The listing builds one solid part. Answer for the finished solid, in the listing's coordinates (mm). Round coordinates to 2 decimals unless told otherwise and drop trailing zeros. Write each loop counter-clockwise with the first axis right and the second up, starting at its lowest first coordinate (ties: lowest second). Pieces come first, ordered by that corner, then holes. Notation, with made-up numbers: M -23,-2 L 2,-2 A12 ccw 2,7 Z; hole C -9.5,4.25 d6. An arc over 180 degrees is marked long. Write each question's results on one line, items separated by ' | '.
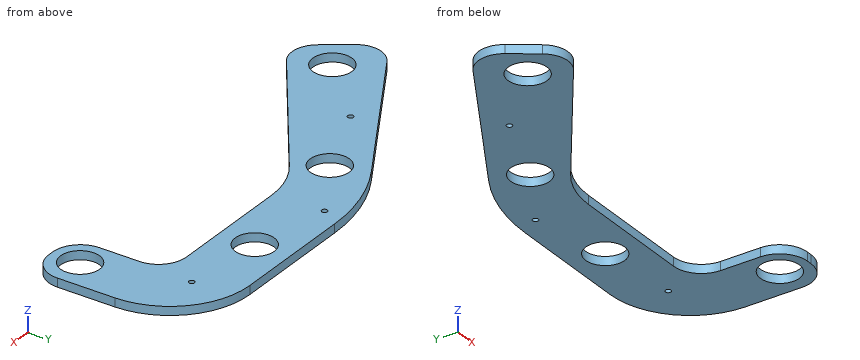
from build123d import *

# Parameters (mm, degrees)
BOSS_EXTRUDE1_DEPTH = 3.175
FILLET4_R           = 127
FILLET8_R           = 6.35
SKETCH4_R           = 14.2875
SKETCH4_R_2         = 2.032
CUT_EXTRUDE1_DEPTH  = 18.415
FILLET20_R          = 33.02
BOSS_EXTRUDE3_DEPTH = 6.35
FILLET23_R          = 127
FILLET24_R          = 19.05
FILLET25_R          = 19.05
SKETCH4_2_R         = 14.2875
SKETCH4_2_R_2       = 2.032
CUT_EXTRUDE2_DEPTH  = 6.35
FILLET27_R          = 60.96
FILLET28_R          = 20.32
FILLET29_R          = 20.32
FILLET30_R          = 20.32
FILLET31_R          = 58.42


with BuildPart() as part:
    # Sketch1 → Boss-Extrude1 (new body)
    with BuildSketch(Plane.XY):
        Polygon((0, 0), (-134.680588616, -95.49423569), (-170.699937974, -44.69423569), (-8.460282393, 50.869520386), (174.726114012, 50.869520386), (174.726114012, -31.75), (174.726114012, -69.85), (130.175, -69.85), (130.175, 0), align=None)
    extrude(amount=BOSS_EXTRUDE1_DEPTH)

    # Fillet4
    fillet4_edges = [part.edges().sort_by_distance(p)[0] for p in [
        (-8.460282393, 50.869520386, 1.5875),
    ]]
    fillet(fillet4_edges, radius=FILLET4_R)

    # Fillet8
    fillet8_edges = [part.edges().sort_by_distance(p)[0] for p in [
        (174.726114012, 50.869520386, 1.5875),
    ]]
    fillet(fillet8_edges, radius=FILLET8_R)

    # Sketch4 → Cut-Extrude1 (cut)
    with BuildSketch(Plane(origin=(0, 0, 0), x_dir=(-1, 0, 0), z_dir=(0, 0, -1))):
        with Locations((-151.503295524, -49.024477041)):
            Circle(SKETCH4_R)
        with Locations((130.843837195, -58.984690885)):
            Circle(SKETCH4_R)
        with Locations((30.055030467, 8.563007376)):
            Circle(SKETCH4_R)
        with Locations((-74.112358802, 25.4)):
            Circle(SKETCH4_R)
        with Locations((85.728358398, -14.612108422)):
            Circle(SKETCH4_R_2)
        with Locations((-132.677584994, 19.676786483)):
            Circle(SKETCH4_R_2)
        with Locations((-16.730295544, 36.917955745)):
            Circle(SKETCH4_R_2)
    extrude(amount=-CUT_EXTRUDE1_DEPTH, mode=Mode.SUBTRACT)

    # Fillet20
    fillet20_edges = [part.edges().sort_by_distance(p)[0] for p in [
        (-134.680588616, -95.49423569, 1.5875),
    ]]
    fillet(fillet20_edges, radius=FILLET20_R)

    # Sketch1<3> → Boss-Extrude3 (add)
    with BuildSketch(Plane.XY):
        Polygon((0, 0), (-134.680588616, -95.49423569), (-170.699937974, -44.69423569), (-8.460282393, 50.869520386), (174.726114012, 50.869520386), (174.726114012, -31.75), (174.726114012, -69.85), (130.175, -69.85), (130.175, 0), align=None)
    extrude(amount=BOSS_EXTRUDE3_DEPTH)

    # Fillet23
    fillet23_edges = [part.edges().sort_by_distance(p)[0] for p in [
        (-8.460282393, 50.869520386, 3.175),
    ]]
    fillet(fillet23_edges, radius=FILLET23_R)

    # Fillet24
    fillet24_edges = [part.edges().sort_by_distance(p)[0] for p in [
        (-170.699937974, -44.69423569, 3.175),
    ]]
    fillet(fillet24_edges, radius=FILLET24_R)

    # Fillet25
    fillet25_edges = [part.edges().sort_by_distance(p)[0] for p in [
        (-134.680588616, -95.49423569, 3.175),
    ]]
    fillet(fillet25_edges, radius=FILLET25_R)

    # Sketch4<2> → Cut-Extrude2 (cut)
    with BuildSketch(Plane(origin=(0, 0, 0), x_dir=(-1, 0, 0), z_dir=(0, 0, -1))):
        with Locations((-151.503295524, -49.024477041)):
            Circle(SKETCH4_2_R)
        with Locations((130.843837195, -58.984690885)):
            Circle(SKETCH4_2_R)
        with Locations((30.055030467, 8.563007376)):
            Circle(SKETCH4_2_R)
        with Locations((-74.112358802, 25.4)):
            Circle(SKETCH4_2_R)
        with Locations((85.728358398, -14.612108422)):
            Circle(SKETCH4_2_R_2)
        with Locations((-132.677584994, 19.676786483)):
            Circle(SKETCH4_2_R_2)
        with Locations((-16.730295544, 36.917955745)):
            Circle(SKETCH4_2_R_2)
    extrude(amount=-CUT_EXTRUDE2_DEPTH, mode=Mode.SUBTRACT)

    # Fillet27
    fillet27_edges = [part.edges().sort_by_distance(p)[0] for p in [
        (0, 0, 3.175),
    ]]
    fillet(fillet27_edges, radius=FILLET27_R)

    # Fillet28
    fillet28_edges = [part.edges().sort_by_distance(p)[0] for p in [
        (130.175, 0, 3.175),
    ]]
    fillet(fillet28_edges, radius=FILLET28_R)

    # Fillet29
    fillet29_edges = [part.edges().sort_by_distance(p)[0] for p in [
        (130.175, -69.85, 3.175),
    ]]
    fillet(fillet29_edges, radius=FILLET29_R)

    # Fillet30
    fillet30_edges = [part.edges().sort_by_distance(p)[0] for p in [
        (174.726114012, -69.85, 3.175),
    ]]
    fillet(fillet30_edges, radius=FILLET30_R)

    # Fillet31
    fillet31_edges = [part.edges().sort_by_distance(p)[0] for p in [
        (174.726114012, 50.869520386, 3.175),
    ]]
    fillet(fillet31_edges, radius=FILLET31_R)


solid = part.part
1) Section D-D (y = 4) is taken. Determine the outline of the cut face in (x, z), then the cut area to 3 significant figures.
Return value:
outline: M -88.03,0 L -43.59,0 L -43.59,6.35 L -88.03,6.35 Z; M -16.52,0 L 173.57,0 L 173.57,6.35 L -16.52,6.35 Z | area: 1,490 mm²
2) Section C-C (z = 3.5) is taken. State how many separate pieces and enclosed holes the cut face has, then the cut area to 3 significant figures.
Return value:
separate pieces: 1 | enclosed holes: 7 | area: 18,200 mm²
3) Section A-A (x = -24.5) is taken. Determine the outline of the cut face in (y, z), then the cut area to 3 significant figures.
Return value:
outline: M -17.37,0 L -4.6,0 L -4.6,6.35 L -17.37,6.35 Z; M 21.73,0 L 40.33,0 L 40.33,6.35 L 21.73,6.35 Z | area: 199 mm²
4) Each of these flat-tipped pins is pushed along its axis until it touches: pin 1 (1.2 mm diameter, centred on x = 152.5, z = 1.5, fed in from -Y); pin 2 (1.9 mm diameter, centred on y = -31, z = 3.5, fed in from -X). Where does it stop, or does it pass through?
Return value:
pin 1: y = -69.85 | pin 2: x = -149.06
5) Find the intervals of material crossed by line 1 (X direction, y = 14, z = 5); line 2 (Y direction, x = 92, z = 3.25); line 3 (Y direction, x = 62, z = 3), in increasing order.
Return value:
line 1: -71.05 to -43.27, -16.84 to 65.5, 82.72 to 170.61 | line 2: 0 to 50.87 | line 3: 0 to 17.82, 32.98 to 50.87
6) Section B-B (y = -40) is taken. Determine the outline of the cut face in (x, z) (3 decimals), then the cut area to 3 significant figures.
Return value:
outline: M -159.006,0 L -56.414,0 L -56.414,6.35 L -159.006,6.35 Z; M 130.175,0 L 140.427,0 L 140.427,6.35 L 130.175,6.35 Z; M 162.58,0 L 174.726,0 L 174.726,6.35 L 162.58,6.35 Z | area: 794 mm²
